Geometry: final body of the model. Coordinates: model frame, mm. A direction names the side the tool comes from. Give positions to 0.01 mm unless a question says otherwise; leave off trailing zeros. Loops run counter-clockwise (first coordinate to the right, second up) from the corner with the lowest first, then second, coordinate; pieces in that order, holes last. Notation, with made-up numbers: (76.25, -21) -> (83.25, -21) arc R32 ccw to (83.25, 6) -> close; hole circle Ø10 at (78, -23.5). An arc over 180 degrees is marked (long way). One line per question, with ' | ' between items. Start each with the question number.
Item 1: Set-up query: faces 3 (the flat face through (-12, 0, 7)), 4 (the flat face through (-0.8, 2, 6)). Return all of +Z, -Z, +X, -X, +Y, -Y with unobstructed straight access to the full face (end or side cutting, diameter ignored); none if empty.
Item 2: Mould query, pull axis Y, two halves, no side actions, for faces 1 (the flat face through (-2.25, 2, 7)), 2 (the flat face through (0, 0, 0)). Classes: released by +Y, released by -Y, zero draft, split by the parting line, or undercut.
Item 3: Pin query (flat end, axial travel): P1, Ø0.7, axis at x = -3.5, y = 2, coming from the +Z side; P2, Ø1, axis at x = -7.5, y = -3.5, coming from the +Z side. Return the tip coordinate at first contact, or that it passes through.
Item 4: Section A-A on z = 8. Return loops of the section in (x, y).
Item 5: Section D-D on y = -1.5. Return loops of the section in (x, z).
Item 6: Section B-B on y = -5.75. Return loops of the section in (x, z), then the cut area to 3 significant figures.
Item 7: Section C-C on x = 7.75. Return loops of the section in (y, z).
Item 8: Material intervals for line 1 along X through (y, z) = (1.75, 4.5); line 2 along Y through (x, z) = (-1.5, 7); line 3 along Y through (x, z) = (-3, 10.5), sorted ascending. Write a range as [from, to].
from build123d import *

# Parameters (mm, degrees)
SKETCH1_W           = 24
SKETCH1_H           = 18
BOSS_EXTRUDE1_DEPTH = 13
FILLET1_R           = 0.35
FILLET2_R           = 0.35
SKETCH2_W           = 23
SKETCH2_H           = 17
CUT_EXTRUDE1_DEPTH  = 11.5
SKETCH11_W          = 4.4
SKETCH11_H          = 6
BOSS_EXTRUDE4_DEPTH = 10
SKETCH12_W          = 4.4
SKETCH12_H          = 1.5
CUT_EXTRUDE6_DEPTH  = 10
SKETCH13_W          = 1.5
SKETCH13_H          = 4.4
CUT_EXTRUDE7_DEPTH  = 10


with BuildPart() as part:
    # Sketch1 → Boss-Extrude1 (new body)
    with BuildSketch(Plane.XY):
        Rectangle(SKETCH1_W, SKETCH1_H)
    extrude(amount=BOSS_EXTRUDE1_DEPTH)

    # Fillet1
    fillet1_edges = [part.edges().sort_by_distance(p)[0] for p in [
        (0, -9, 0),
        (-12, 0, 0),
        (0, 9, 0),
        (12, 0, 0),
    ]]
    fillet(fillet1_edges, radius=FILLET1_R)

    # Fillet2
    # the kernel refuses this fillet: 0.35 mm, written as the material it takes off along each edge
    with BuildSketch(Plane(origin=(11.65, 8.65, 0.35), x_dir=(0, 1, 0), z_dir=(1, 0, 0))) as fillet2_piece_1_section:
        Polygon((0, 0), (FILLET2_R, 0), (FILLET2_R, -FILLET2_R), (0, -FILLET2_R), align=None)
    fillet2_piece_1 = extrude(amount=FILLET2_R, mode=Mode.PRIVATE)
    fillet2_piece_1 = fillet2_piece_1 - Plane(origin=(11.65, 8.65, 0.35), x_dir=(0, -0.7071067811865475, 0.7071067811865475), z_dir=(1, 0, 0)) * Sphere(FILLET2_R, mode=Mode.PRIVATE)
    add(fillet2_piece_1, mode=Mode.SUBTRACT)
    with BuildSketch(Plane(origin=(11.65, -8.65, 0.35), x_dir=(1, 0, 0), z_dir=(0, -1, 0))) as fillet2_piece_2_section:
        Polygon((0, 0), (FILLET2_R, 0), (FILLET2_R, -FILLET2_R), (0, -FILLET2_R), align=None)
    fillet2_piece_2 = extrude(amount=FILLET2_R, mode=Mode.PRIVATE)
    fillet2_piece_2 = fillet2_piece_2 - Plane(origin=(11.65, -8.65, 0.35), x_dir=(-0.7071067811865475, 0, 0.7071067811865475), z_dir=(0, -1, 0)) * Sphere(FILLET2_R, mode=Mode.PRIVATE)
    add(fillet2_piece_2, mode=Mode.SUBTRACT)
    with BuildSketch(Plane(origin=(-11.65, 8.65, 0.35), x_dir=(0, 1, 0), z_dir=(-1, 0, 0))) as fillet2_piece_3_section:
        Polygon((0, 0), (FILLET2_R, 0), (FILLET2_R, FILLET2_R), (0, FILLET2_R), align=None)
    fillet2_piece_3 = extrude(amount=FILLET2_R, mode=Mode.PRIVATE)
    fillet2_piece_3 = fillet2_piece_3 - Plane(origin=(-11.65, 8.65, 0.35), x_dir=(0, -0.7071067811865475, 0.7071067811865475), z_dir=(-1, 0, 0)) * Sphere(FILLET2_R, mode=Mode.PRIVATE)
    add(fillet2_piece_3, mode=Mode.SUBTRACT)
    with BuildSketch(Plane(origin=(-11.65, -8.65, 0.35), x_dir=(-1, 0, 0), z_dir=(0, -1, 0))) as fillet2_piece_4_section:
        Polygon((0, 0), (FILLET2_R, 0), (FILLET2_R, FILLET2_R), (0, FILLET2_R), align=None)
    fillet2_piece_4 = extrude(amount=FILLET2_R, mode=Mode.PRIVATE)
    fillet2_piece_4 = fillet2_piece_4 - Plane(origin=(-11.65, -8.65, 0.35), x_dir=(0.7071067811865475, 0, 0.7071067811865475), z_dir=(0, -1, 0)) * Sphere(FILLET2_R, mode=Mode.PRIVATE)
    add(fillet2_piece_4, mode=Mode.SUBTRACT)
    with BuildSketch(Plane(origin=(12, -9, 0.35), x_dir=(-1, 0, 0), z_dir=(0, 0, 1)), Plane(origin=(12, 9, 0.35), x_dir=(0, -1, 0), z_dir=(0, 0, 1))) as fillet2_piece_5:
        with BuildLine():
            CenterArc((FILLET2_R, -FILLET2_R), FILLET2_R, 90, 90)
            Line((0, -FILLET2_R), (0, 0))
            Line((0, 0), (FILLET2_R, 0))
        make_face()
    extrude(amount=13.525, mode=Mode.SUBTRACT)
    with BuildSketch(Plane(origin=(-12, -9, 0.35), x_dir=(1, 0, 0), z_dir=(0, 0, 1)), Plane(origin=(-12, 9, 0.35), x_dir=(0, -1, 0), z_dir=(0, 0, 1))) as fillet2_piece_6:
        with BuildLine():
            CenterArc((FILLET2_R, FILLET2_R), FILLET2_R, 180, 90)
            Line((0, FILLET2_R), (0, 0))
            Line((0, 0), (FILLET2_R, 0))
        make_face()
    extrude(amount=13.525, mode=Mode.SUBTRACT)

    # Sketch2 → Cut-Extrude1 (cut)
    with BuildSketch(Plane.XY.offset(13)):
        Rectangle(SKETCH2_W, SKETCH2_H)
    extrude(amount=-CUT_EXTRUDE1_DEPTH, mode=Mode.SUBTRACT)

    # Sketch11 → Boss-Extrude4 (add)
    with BuildSketch(Plane.XY.offset(1.5)):
        with Locations((-3, 0)):
            Rectangle(SKETCH11_W, SKETCH11_H)
    extrude(amount=BOSS_EXTRUDE4_DEPTH)

    # Sketch12 → Cut-Extrude6 (cut)
    with BuildSketch(Plane.XY.offset(11.5)):
        with Locations((-3, 0.045549291)):
            Rectangle(SKETCH12_W, SKETCH12_H)
    extrude(amount=-CUT_EXTRUDE6_DEPTH, mode=Mode.SUBTRACT)

    # Sketch13 → Cut-Extrude7 (cut)
    with BuildSketch(Plane.XY.offset(11.5)):
        with Locations((-3, 0.045549291)):
            Rectangle(SKETCH13_W, SKETCH13_H)
    extrude(amount=-CUT_EXTRUDE7_DEPTH, mode=Mode.SUBTRACT)


solid = part.part
Result sheet:
1) face 3: +Z, -Z, -X, +Y, -Y | face 4: +Z
2) face 1: undercut | face 2: zero draft
3) P1: stops at z = 11.5 | P2: stops at z = 1.5
4) outline: (-12, -8.65) arc R0.35 ccw to (-11.65, -9) -> (11.65, -9) arc R0.35 ccw to (12, -8.65) -> (12, 8.65) arc R0.35 ccw to (11.65, 9) -> (-11.65, 9) arc R0.35 ccw to (-12, 8.65) -> close; (-5.2, -3) -> (-0.8, -3) -> (-0.8, -0.7) -> (-2.25, -0.7) -> (-2.25, -2.15) -> (-3.75, -2.15) -> (-3.75, -0.7) -> (-5.2, -0.7) -> close; (-5.2, 0.8) -> (-3.75, 0.8) -> (-3.75, 2.25) -> (-2.25, 2.25) -> (-2.25, 0.8) -> (-0.8, 0.8) -> (-0.8, 3) -> (-5.2, 3) -> close; hole (-11.5, -8.5) -> (11.5, -8.5) -> (11.5, 8.5) -> (-11.5, 8.5) -> close
5) outline: (-12, 0.35) arc R0.35 ccw to (-11.65, 0) -> (11.65, 0) arc R0.35 ccw to (12, 0.35) -> (12, 13) -> (11.5, 13) -> (11.5, 1.5) -> (-0.8, 1.5) -> (-0.8, 11.5) -> (-2.25, 11.5) -> (-2.25, 1.5) -> (-3.75, 1.5) -> (-3.75, 11.5) -> (-5.2, 11.5) -> (-5.2, 1.5) -> (-11.5, 1.5) -> (-11.5, 13) -> (-12, 13) -> close
6) outline: (-12, 0.35) arc R0.35 ccw to (-11.65, 0) -> (11.65, 0) arc R0.35 ccw to (12, 0.35) -> (12, 13) -> (11.5, 13) -> (11.5, 1.5) -> (-11.5, 1.5) -> (-11.5, 13) -> (-12, 13) -> close | area: 47.4 mm²
7) outline: (-9, 0.35) arc R0.35 ccw to (-8.65, 0) -> (8.65, 0) arc R0.35 ccw to (9, 0.35) -> (9, 13) -> (8.5, 13) -> (8.5, 1.5) -> (-8.5, 1.5) -> (-8.5, 13) -> (-9, 13) -> close
8) line 1: x = [-12, -11.5], [-5.2, -3.75], [-2.25, -0.8], [11.5, 12] | line 2: y = [-9, -8.5], [-3, -0.7], [0.8, 3], [8.5, 9] | line 3: y = [-9, -8.5], [-3, -2.15], [2.25, 3], [8.5, 9]
